```python
from build123d import *

# Parameters (mm, degrees)
SKETCH1_R           = 6
BOSS_EXTRUDE1_DEPTH = 4.7625
FILLET1_R           = 5


with BuildPart() as part:
    # Sketch1 → Boss-Extrude1 (new body)
    with BuildSketch(Plane(origin=(0, 0, 0), x_dir=(1, 0, 0), z_dir=(0, 1, 0))):
        Polygon((0, -11.25), (0, 11.25), (-30, 7.5), (-30, -7.5), align=None)
        with Locations((-20, 0)):
            Circle(SKETCH1_R, mode=Mode.SUBTRACT)
    extrude(amount=BOSS_EXTRUDE1_DEPTH)

    # Fillet1
    fillet1_edges = [part.edges().sort_by_distance(p)[0] for p in [
        (-30, 2.38125, 7.5),
        (-30, 2.38125, -7.5),
    ]]
    fillet(fillet1_edges, radius=FILLET1_R)


solid = part.part
```
Check sheet for the modelled part. Datum: model origin and axes. Units: mm. Round coordinates to 2 decimals unless told otherwise and drop trailing zeros. Order: outer loops, then holes, each group sorted by start corner. A loop starts at its lowest first (then second) coordinate and runs counter-clockwise, first axis right, second up. Notation, with made-up numbers: (-31, 40) -> (-23, 40) arc R33 cw to (-23, 78) -> close; hole circle Ø7 at (82.25, -5). An arc over 180 degrees is marked (long way). Use CSV: the item, a comma, the result in double quotes.
(1) Cross-section at B-B (z = 0). Record the boundary of the cut face in (x, y).
Worked out:
outline,"(-30, 0) -> (-26, 0) -> (-26, 4.76) -> (-30, 4.76) -> close; (-14, 0) -> (0, 0) -> (0, 4.76) -> (-14, 4.76) -> close"
(2) Material ranges on line 1 along X through (y, z) = (4.2, 0); line 2 along X through (y, z) = (3.95, -3); line 3 along Z through (x, y) = (-20, 2), recorded low to high. Write a range as from..to.
Worked out:
line 1,"-30..-26, -14..0"
line 2,"-30..-25.2, -14.8..0"
line 3,"-8.75..-6, 6..8.75"
(3) Cross-section at D-D (z = -9.5). Record the boundary of the cut face in (x, y), and give its area (3 significant figures).
Worked out:
outline,"(-14, 0) -> (0, 0) -> (0, 4.76) -> (-14, 4.76) -> close"
area,"66.7 mm²"
(4) Draft check along Z on faces 1 (the face through (-24.76, 2.35, 3.65)), 2 (the face through (-12.63, 2.35, -9.67)), 3 (the face through (0, 2, 0)), 4 (the face through (-28.715, 2.415, 6.433)). Enter one of: pulls with the +Z half, pulls with the -Z half, needs draft (parallel to the pull), parting line crosses it, or undercut.
Worked out:
face 1,"undercut"
face 2,"pulls with the -Z half"
face 3,"needs draft"
face 4,"pulls with the +Z half"
(5) Depth check by flat-ended pin: pin 1 (1.5 mm diameter, centred on x = -3.5, y = 2, fed in from -Z); pin 2 (2 mm diameter, centred on x = -8.5, y = 3, fed in from +Z). Enter the tip coordinate at first touch or a pass-through.
Worked out:
pin 1,"z = -10.91"
pin 2,"z = 10.31"
(6) Cross-section at A-A (x = -20). Record the boundary of the cut face in (y, z).
Worked out:
outline,"(0, -8.75) -> (4.76, -8.75) -> (4.76, -6) -> (0, -6) -> close; (0, 6) -> (4.76, 6) -> (4.76, 8.75) -> (0, 8.75) -> close"
(7) Cross-section at C-C (y = 1.25). Record the boundary of the cut face in (x, z), and give its area (3 significant figures).
Worked out:
outline,"(-30, -3.09) arc R5 ccw to (-25.62, -8.05) -> (0, -11.25) -> (0, 11.25) -> (-25.62, 8.05) arc R5 ccw to (-30, 3.09) -> close; hole circle Ø12 at (-20, 0)"
area,"441 mm²"
